```python
from build123d import *

# Parameters (mm, degrees)
FILLET1_R   = 0.1
HEX_2_DEPTH = 1.2


with BuildPart() as part:
    # BodySke → BaseBody (revolve)
    with BuildSketch(Plane.XY):
        Polygon((0, 0), (0, 2.85), (0.35, 2.85), (1.7, 1.5), (15.7195, 1.5), (16, 1.2195), (16, 0), align=None)
    revolve(axis=Axis((0, 0, 0), (1, 0, 0)))

    # Fillet1
    fillet1_edges = [part.edges().sort_by_distance(p)[0] for p in [
        (1.7, -1.5, 0),
    ]]
    fillet(fillet1_edges, radius=FILLET1_R)

    # Sketch2 → PreBroach (revolve, cut)
    with BuildSketch(Plane.XY):
        Polygon((0, 1.01), (1.2, 1.01), (1.783123772, 0), (0, 0), align=None)
    revolve(axis=Axis((0, 0, 0), (1, 0, 0)), mode=Mode.SUBTRACT)

    # Sketch3 → Hex 2 (cut)
    with BuildSketch(Plane.ZY):
        Polygon((-1.01, -0.583123772), (-1.01, 0.583123772), (0, 1.166247544), (1.01, 0.583123772), (1.01, -0.583123772), (0, -1.166247544), align=None)
    extrude(amount=-HEX_2_DEPTH, mode=Mode.SUBTRACT)


solid = part.part
```
Input: part model. Units: mm. Frame: model coordinates. A direction names the side the tool comes from. Coordinates: 2 decimals unless noted, no trailing zeros. Write each loop counter-clockwise with the first axis right and the second up, starting at its lowest first coordinate (ties: lowest second). Pieces come first, ordered by that corner, then holes. Notation, with made-up numbers: (51, 87.25) -> (62, 87.25) arc R5 ccw to (62, 94.25) -> close; hole circle Ø10 at (82.25, 61). An arc over 180 degrees is marked (long way). Answer as a JSON object with one key per item and string values.
1. Access query for faces 1 (the face through (8.83, -1.5, 0.07)), 2 (the face through (16, 0, 0)), 3 (the face through (0.592, -0.879, -0.498)). Directions: +Z, -Z, +X, -X, +Y, -Y. A direction counts if a zero-diameter tool reaches every point of the face in a straight line with its end or side. Return the directions, or none.
Result set:
{"face 1": "+X", "face 2": "+Z, -Z, +X, +Y, -Y", "face 3": "-X"}
2. Material intervals for line 1 (X direction, y = 1.2, z = 1.4); line 2 (Y direction, x = 2.5, z = 1.1); line 3 (Z direction, x = 2, y = 1.15), sorted ascending. Write a range as from..to.
Result set:
{"line 1": "x = 0..1.36", "line 2": "y = -1.02..1.02", "line 3": "z = -0.96..0.96"}
3. First-contact query: P1, Ø1, axis at x = 10, z = 0, coming from the -Y side; P2, Ø1.5, axis at x = 5.5, y = 0, coming from the -Z side. Flat tips, straight axial feed; report the tip coordinate or a pass-through.
Result set:
{"P1": "stops at y = -1.5", "P2": "stops at z = -1.5"}
4. Mould query, pull axis Z, two halves, no side actions, for faces 4 (the face through (1, 0, -1.01)), 5 (the face through (0.177, -2.262, -1.734)), 6 (the face through (0, 0, -1.2)). Classes: released by +Z, released by -Z, zero draft, split by the parting line, or undercut.
Result set:
{"face 4": "undercut", "face 5": "split by the parting line", "face 6": "zero draft"}
5. Section A-A on x = 7.5. Return the cut outline in (y, z), then the cut area to 3 significant figures.
Result set:
{"outline": "circle Ø3 at (0, 0)", "area": "7.07 mm2"}
